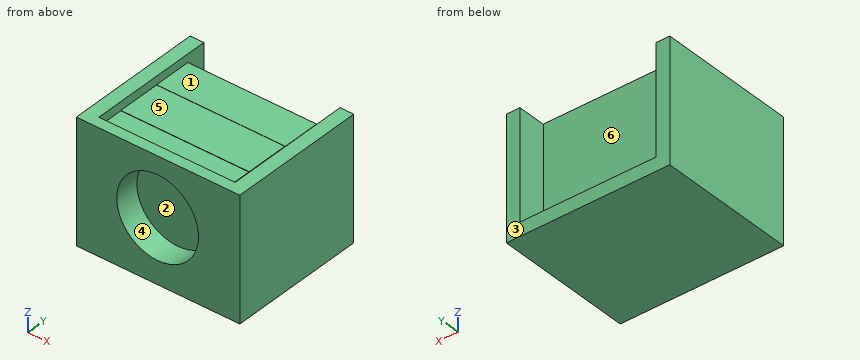
from build123d import *

# Parameters (mm, degrees)
SKETCH1_W           = 500
SKETCH1_H           = 400
BOSS_EXTRUDE2_DEPTH = 510
SKETCH2_W           = 500
SKETCH2_H           = 400
CUT_EXTRUDE1_DEPTH  = 470
SKETCH4_W           = 470
SKETCH4_H           = 370
BOSS_EXTRUDE5_DEPTH = 80
SKETCH6_W           = 470.959249671
SKETCH6_H           = 371.189101319
BOSS_EXTRUDE7_DEPTH = 160
SKETCH7_W           = 472.653238371
SKETCH7_H           = 372.039567124
BOSS_EXTRUDE8_DEPTH = 140
SKETCH8_R           = 150
CUT_EXTRUDE2_DEPTH  = 90


with BuildPart() as part:
    # Sketch1 → Boss-Extrude2 (new body)
    with BuildSketch(Plane(origin=(0, 0, 0), x_dir=(1, 0, 0), z_dir=(0, 1, 0))):
        Polygon((-248.47715736, 234.517766497), (-298.47715736, 234.517766497), (-298.47715736, 184.517766497), (-298.47715736, -215.482233503), (-248.47715736, -215.482233503), (-248.47715736, 184.517766497), (251.52284264, 184.517766497), (251.52284264, -215.482233503), (301.52284264, -215.482233503), (301.52284264, 184.517766497), (301.52284264, 234.517766497), (251.52284264, 234.517766497), align=None)
        with Locations((1.52284264, -15.482233503)):
            Rectangle(SKETCH1_W, SKETCH1_H)
    extrude(amount=BOSS_EXTRUDE2_DEPTH)

    # Sketch2 → Cut-Extrude1 (cut)
    with BuildSketch(Plane(origin=(0, 510, 0), x_dir=(1, 0, 0), z_dir=(0, 1, 0))):
        with Locations((1.52284264, -15.482233503)):
            Rectangle(SKETCH2_W, SKETCH2_H)
    extrude(amount=-CUT_EXTRUDE1_DEPTH, mode=Mode.SUBTRACT)

    # Sketch4 → Boss-Extrude5 (add)
    with BuildSketch(Plane(origin=(0, 40, 0), x_dir=(1, 0, 0), z_dir=(0, 1, 0))):
        with Locations((1.52284264, -15.482233503)):
            Rectangle(SKETCH4_W, SKETCH4_H)
    extrude(amount=BOSS_EXTRUDE5_DEPTH)

    # Sketch6 → Boss-Extrude7 (add)
    with BuildSketch(Plane(origin=(0, 120, 0), x_dir=(1, 0, 0), z_dir=(0, 1, 0))):
        with Locations((2.002467475, -16.076784163)):
            Rectangle(SKETCH6_W, SKETCH6_H)
    extrude(amount=BOSS_EXTRUDE7_DEPTH)

    # Sketch7 → Boss-Extrude8 (add)
    with BuildSketch(Plane(origin=(0, 280, 0), x_dir=(1, 0, 0), z_dir=(0, 1, 0))):
        with Locations((2.849461826, -16.502017065)):
            Rectangle(SKETCH7_W, SKETCH7_H)
    extrude(amount=BOSS_EXTRUDE8_DEPTH)

    # Sketch8 → Cut-Extrude2 (cut)
    with BuildSketch(Plane.XZ):
        with Locations(Location((0, 0, 0), (0, 0, 270))):
            Circle(SKETCH8_R)
    extrude(amount=-CUT_EXTRUDE2_DEPTH, mode=Mode.SUBTRACT)


solid = part.part
CAD build for the part. Positions are in the model's coordinates, mm. Face numbers are marked on the shaded views. A direction names the side the tool comes from. Give positions to 0.01 mm unless a question says otherwise; leave off trailing zeros. Loops run counter-clockwise (first coordinate to the right, second up) from the corner with the lowest first, then second, coordinate; pieces in that order, holes last. Notation, with made-up numbers: M 8.25,85.5 L 32.25,85.5 A21 ccw 32.25,99.5 Z; hole C 39.25,63.5 d5. An arc over 180 degrees is marked long. One line per question, with ' | ' between items. Start each with the question number.
1. Saw through at B-B on z = 0. Give the cut face in (x, y), plus the area to 3 significant figures.
2. Saw through at D-D on y = 448.5. Give the cut face in (x, z), plus the area to 3 significant figures.
3. Probe L1, parallel to X at y = 418, z = 80; L2, parallel to X at y = 271.5, z = 57; L3, parallel to Z at x = 10.5, y = 351.5. List the from-to ranges inside material, lowest first. Write a range as from..to.
4. Saw through at C-C on x = 0. Give the cut face in (y, z).
5. Two-plate mould, pull along Y, no slides. Class the marked faces 4, 5 and 6: pulls with the +Y half, pulls with the -Y half, needs draft (parallel to the pull), parting line crosses it, or undercut.
6. Flat gauge pins, fed straight in: pin 1 (5 mm diameter, centred on x = -221, y = 211, fed in from +Z); pin 2 (4 mm diameter, centred on x = -25.5, z = -41, fed in from -Y); pin 3 (12 mm diameter, centred on x = 112, y = 305.5, fed in from +Z). Where does each tip first touch, or does it go through?
7. Saw through at A-A on y = 143.5. Give the cut face in (x, z).
8. 3-axis set-ups, long thin cutter, end or side, ignore diameter. For the marked faces 1, 2 and 3: which of +Z, -Z, +X, -X, +Y, -Y reach the whole face in a straight line?
Result sheet:
1) outline: M -298.48,0 L -150,0 L -150,90 L 150,90 L 150,0 L 301.52,0 L 301.52,510 L 251.52,510 L 251.52,40 L 236.52,40 L 236.52,120 L 237.48,120 L 237.48,280 L 239.18,280 L 239.18,420 L -233.48,420 L -233.48,40 L -248.48,40 L -248.48,510 L -298.48,510 Z | area: 223,000 mm^2
2) outline: M -298.48,-234.52 L 301.52,-234.52 L 301.52,215.48 L 251.52,215.48 L 251.52,-184.52 L -248.48,-184.52 L -248.48,215.48 L -298.48,215.48 Z | area: 70,000 mm^2
3) L1: x = -298.48..-248.48, -233.48..239.18, 251.52..301.52 | L2: x = -298.48..-248.48, -233.48..237.48, 251.52..301.52 | L3: z = -234.52..-184.52, -169.52..202.52
4) outline: M 0,-234.52 L 510,-234.52 L 510,-184.52 L 40,-184.52 L 40,-169.52 L 420,-169.52 L 420,202.52 L 280,202.52 L 280,201.67 L 120,201.67 L 120,200.48 L 40,200.48 L 40,215.48 L 0,215.48 L 0,150 L 90,150 L 90,-150 L 0,-150 Z
5) face 4: needs draft | face 5: undercut | face 6: pulls with the +Y half
6) pin 1: stops at z = 201.67 | pin 2: stops at y = 90 | pin 3: stops at z = 202.52
7) outline: M -298.48,-234.52 L 301.52,-234.52 L 301.52,215.48 L 251.52,215.48 L 251.52,-184.52 L -248.48,-184.52 L -248.48,215.48 L -298.48,215.48 Z; M -233.48,-169.52 L 237.48,-169.52 L 237.48,201.67 L -233.48,201.67 Z
8) face 1: +Z, +Y | face 2: -Y | face 3: +Z, -Z, +X, -X, +Y
